Source: three-view drawing plus pictorial views. Frame: mm from the lowest corner of the part. A direction names the side the tool comes from. Give positions to 0.01 mm unless a question says otherwise; leave off trailing zeros. Order: outer loops, then holes, each group sorted by start corner. A loop starts at its lowest first (then second) coordinate and runs counter-clockwise, first axis right, second up. Notation, with made-up numbers: (57, 80.5) - (74, 80.5) arc R19 ccw to (74, 95.5) - close; hole circle Ø1 at (-32.5, 29). An arc over 180 degrees is marked (long way). Answer in a Markdown table with one row per item. Add a question column.
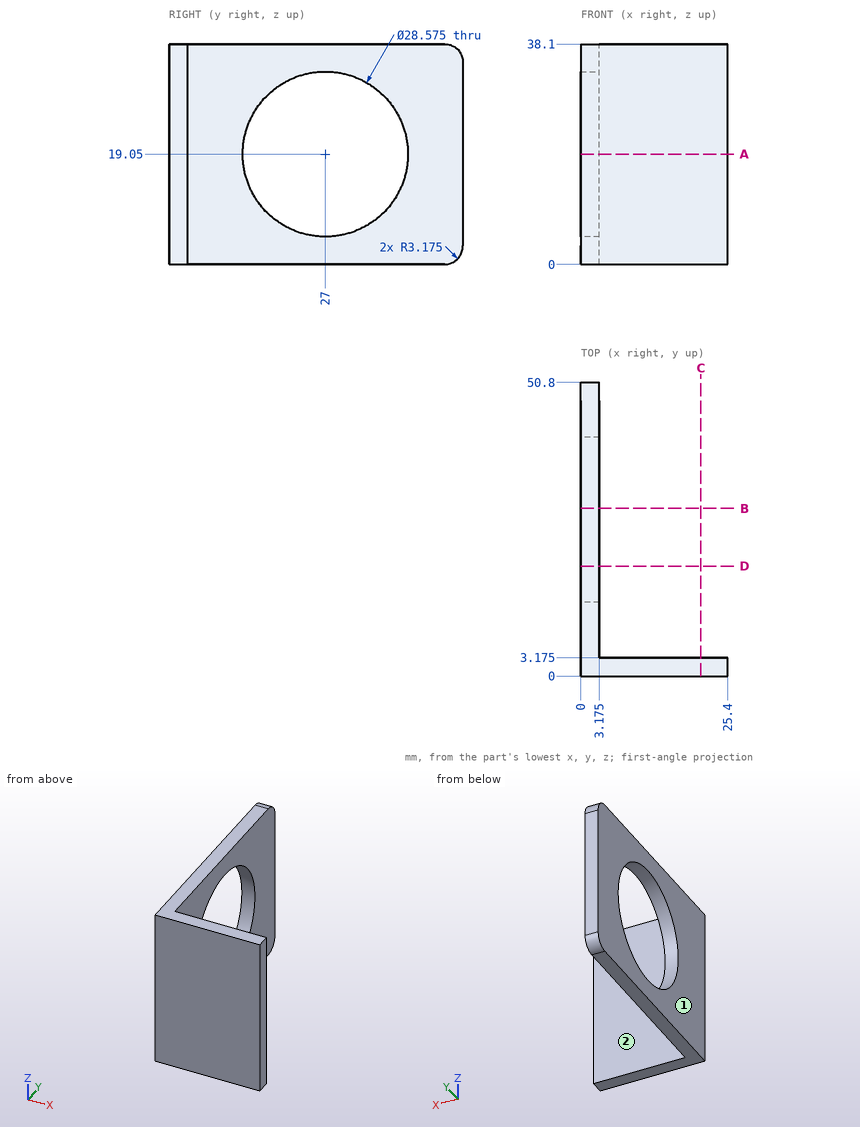
Q1. Line query: probe 1 along Y at (x, z) = (2.3, 19.05); probe 2 along Y at (x, z) = (21.5, 17) (3 decimals); probe 3 along Z at (x, y) = (2.5, 38). Output: solid intervals per line, ascending.
Q2. Section A-A, the plane z = 19.05. Return loops of the section in (x, y) (1 decimal), then the cut area to 3 significant figures.
Q3. Access query for the marked faces 1 and 2. Directions: +Z, -Z, +X, -X, +Y, -Y. A direction counts if a zero-diameter tool reaches every point of the face in a straight line with its end or side. Return the directions, or none.
Q4. Section B-B, the plane y = 29. Return loops of the section in (x, z) (1 decimal).
Q5. Contact query for flat-ended pins moving along their axis: P1, Ø8, axis at x = 16.5, z = 30.5, coming from the -Y side; P2, Ø19, axis at y = 21, z = 13.5, coming from the +X side (3 decimals); P3, Ø12, axis at x = 17.5, z = 16, coming from the +Y side (3 decimals). Output: stop coordinate, or through.
Q6. Section C-C, the plane x = 20.75. Return loops of the section in (y, z) (3 decimals).
Q7. Section D-D, the plane y = 19. Return loops of the section in (x, z) (1 decimal).
Computed:
| question | item | result |
|---|---|---|
| 1 | probe 1 | y = 0 to 12.71, 41.29 to 50.8 |
| 1 | probe 2 | y = 0 to 3.175 |
| 1 | probe 3 | z = 0 to 9.93, 28.17 to 38.1 |
| 2 | outline | (0, 0) - (25.4, 0) - (25.4, 3.2) - (3.2, 3.2) - (3.2, 12.7) - (0, 12.7) - close; (0, 41.3) - (3.2, 41.3) - (3.2, 50.8) - (0, 50.8) - close |
| 2 | area | 141 mm^2 |
| 3 | face 1 | +Z, -Z, -X, +Y, -Y |
| 3 | face 2 | +Z, -Z, +X, +Y |
| 4 | outline | (0, 0) - (3.2, 0) - (3.2, 4.9) - (0, 4.9) - close; (0, 33.2) - (3.2, 33.2) - (3.2, 38.1) - (0, 38.1) - close |
| 5 | P1 | stops at y = 0 |
| 5 | P2 | stops at x = 3.175 |
| 5 | P3 | stops at y = 3.175 |
| 6 | outline | (0, 0) - (3.175, 0) - (3.175, 38.1) - (0, 38.1) - close |
| 7 | outline | (0, 0) - (3.2, 0) - (3.2, 7.2) - (0, 7.2) - close; (0, 30.9) - (3.2, 30.9) - (3.2, 38.1) - (0, 38.1) - close |
